Print and shaded views of the part. All mm, measured from the part's lowest x, y and z. A direction names the side the tool comes from. Round coordinates to 2 decimals unless told otherwise and drop trailing zeros. Loops run counter-clockwise (first coordinate to the right, second up) from the corner with the lowest first, then second, coordinate; pieces in that order, holes last. Notation, with made-up numbers: (86, 18) - (138, 18) arc R8 cw to (138, 22) - close; hole circle Ø11 at (72.5, 82). An arc over 180 degrees is marked (long way). Answer as a JSON object with one key per item and string values.
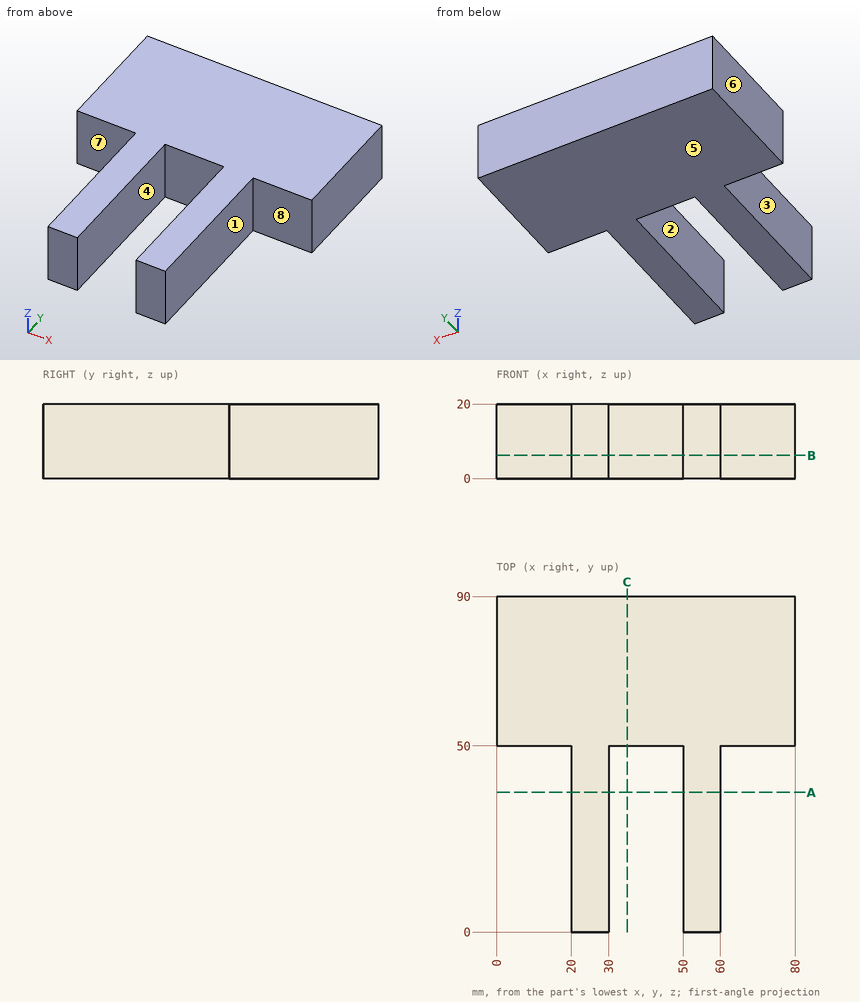
1) Slice it at C-C on x = 35. List the corners of the cut face in (y, z).
Values follow:
{"outline": "(50, 0) - (90, 0) - (90, 20) - (50, 20) - close"}
2) Two-plate mould, pull along X, no slides. Class the marked faces 1, 2 and 3: pulls with the +X half, pulls with the -X half, needs draft (parallel to the pull), parting line crosses it, or undercut.
Values follow:
{"face 1": "pulls with the +X half", "face 2": "undercut", "face 3": "pulls with the -X half"}
3) Slice it at B-B on z = 6.25. List the corners of the cut face in (x, y), then the cut area to 3 significant figures.
Values follow:
{"outline": "(0, 50) - (20, 50) - (20, 0) - (30, 0) - (30, 50) - (50, 50) - (50, 0) - (60, 0) - (60, 50) - (80, 50) - (80, 90) - (0, 90) - close", "area": "4,200 mm²"}
4) Tool access for the marked faces 4, 5, 6, 7 and 8: list every direction of +Z, -Z, +X, -X, +Y, -Y with a clear straight run to the whole face (end or side of a thin tool).
Values follow:
{"face 4": "+Z, -Z, -Y", "face 5": "-Z, +X, -X, +Y, -Y", "face 6": "+Z, -Z, -X, +Y, -Y", "face 7": "+Z, -Z, -X, -Y", "face 8": "+Z, -Z, +X, -Y"}
5) Drop flat-ended pins along their axis: P1, Ø10, axis at y = 37, z = 6, coming from the -X side; P2, Ø10, axis at x = 38.5, z = 5, coming from the -Y side; P3, Ø6, axis at y = 22.5, z = 7.5, coming from the +X side. Give the stop position or say it passes through.
Values follow:
{"P1": "x = 20", "P2": "y = 50", "P3": "x = 60"}
6) Slice it at A-A on y = 37.5. List the corners of the cut face in (x, z).
Values follow:
{"outline": "(20, 0) - (30, 0) - (30, 20) - (20, 20) - close; (50, 0) - (60, 0) - (60, 20) - (50, 20) - close"}
7) Probe probe 1 along X at (y, z) = (48, 2.75); probe 2 along Y at (x, z) = (32, 14). List the from-to ranges inside material, lowest first.
Values follow:
{"probe 1": "20 to 30, 50 to 60", "probe 2": "50 to 90"}
